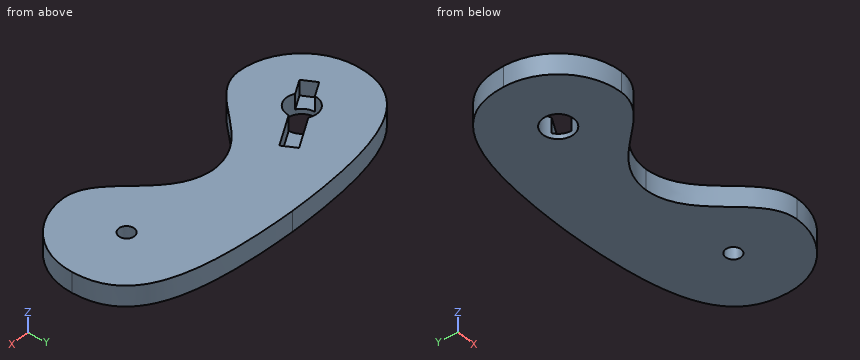
from build123d import *

# Parameters (mm, degrees)
SKETCH_1_R          = 1.5
SKETCH_1_R_2        = 3
EXTRUDE_1_DEPTH     = 4
CUT_EXTRUDE_2_DEPTH = 3


with BuildPart() as part:
    # 草图1 → 凸台-拉伸1 (new body)
    with BuildSketch(Plane.XY):
        with BuildLine():
            ThreePointArc((112.5, 0), (108.838834765, -8.838834765), (100, -12.5))
            add(Edge.make_bspline(
                [(100, -12.5), (92.140208688, -12.329014368), (89.825172612, -0.222632889), (80, 0)],
                knots=[0, 0, 0, 0, 1, 1, 1, 1], degree=3))
            add(Edge.make_bspline(
                [(60, -12.5), (67.859791312, -12.329014368), (70.174827388, -0.222632889), (80, 0)],
                knots=[0, 0, 0, 0, 1, 1, 1, 1], degree=3))
            ThreePointArc((60, -12.5), (51.161165235, -8.838834765), (47.5, 0))
            add(Edge.make_bspline(
                [(47.5, 0), (47.5, 11.115830806), (57.235300252, 15.170917893), (80, 15.396531985)],
                knots=[0, 0, 0, 0, 1, 1, 1, 1], degree=3))
            add(Edge.make_bspline(
                [(112.5, 0), (112.5, 11.115830806), (102.764699748, 15.170917893), (80, 15.396531985)],
                knots=[0, 0, 0, 0, 1, 1, 1, 1], degree=3))
        make_face()
        with Locations((100, 0)):
            Circle(SKETCH_1_R, mode=Mode.SUBTRACT)
        with Locations((60, 0)):
            Circle(SKETCH_1_R_2, mode=Mode.SUBTRACT)
    extrude(amount=EXTRUDE_1_DEPTH)

    # 草图5 → 切除-拉伸2 (cut)
    with BuildSketch(Plane.XY.offset(4)):
        Polygon((54.803847577, -3), (54.053847577, -1.700961894), (67.910254038, 6.299038106), (69.410254038, 3.700961894), (55.553847577, -4.299038106), align=None)
    extrude(amount=-CUT_EXTRUDE_2_DEPTH, mode=Mode.SUBTRACT)


solid = part.part
Check sheet for the modelled part. Datum: model origin and axes. Units: mm. Round coordinates to 2 decimals unless told otherwise and drop trailing zeros.
(1) Scan lines: probe 1 along Y at (x, z) = (66, 1.8); probe 2 along X at (y, z) = (-2.5, 0.35); probe 3 along Y at (x, z) = (60, 3). Record each from-to range of solid material in increasing order.
(2) Go/stop test with flat-tipped pins: P1, Ø5, axis at x = 66.5, y = 3.5, coming from the +Z side; P2, Ø1, axis at y = 12, z = 2.5, coming from the +X side; P3, Ø5.5, axis at x = 60, y = 0, coming from the -Z side; P4, Ø2, axis at y = 3.5, z = 0.5, coming from the +X side. Record where each tip stops, or that it passes through.
(3) Cross-section at A-A, the plane z = 3.15. State how many separate pieces and enclosed holes the cut face has, and give its area (3 significant figures).
Check sheet entries:
1. probe 1: y = -9.7 to 1.73, 5.2 to 14.55
1. probe 2: x = 47.75 to 58.34, 61.66 to 73.17, 86.83 to 112.25
1. probe 3: y = -12.5 to -3, 3 to 13.43
2. P1: stops at z = 4
2. P2: stops at x = 105.37
2. P3: passes through
2. P4: stops at x = 112.32
3. separate pieces: 1
3. enclosed holes: 2
3. area: 1,260 mm2
